For this review, take the finished solid that the model builds, in its own axes (mm). A direction names the side the tool comes from. Coordinates: 2 decimals unless noted, no trailing zeros. Order: outer loops, then holes, each group sorted by start corner. A loop starts at its lowest first (then second) coordinate and runs counter-clockwise, first axis right, second up. Notation, with made-up numbers: (69, -22) -> (120, -22) arc R16 ccw to (120, 6) -> close; hole circle Ø5 at (0.25, -6.5). An arc over 180 degrees is marked (long way). Write item = value, one per line. Start each with the question number.
1) Machinability: for faces 4 (the face through (41, 9, -107.95)), 5 (the face through (45, 53, -295.275)), 6 (the face through (2.053, 67.327, -201.314)), which of the approach directions +Z, -Z, +X, -X, +Y, -Y give a long, thin tool a straight path to every point of the face, cutting with its end or side? Answer none if there is none.
2) Consider section C-C on z = -123. Give the boundary of the cut face in (x, y) (3 decimals).
3) Insertion check: pin 1 Ø10 at (x, y) = (68, 130.5) entering from -Z; pin 2 Ø2.5 at (x, z) = (65.5, -294) entering from +Y (3 decimals); pin 3 Ø12 at (x, z) = (50.5, -200.5) entering from +Y (3 decimals). Each pin has a flat end and moves straight along its axis. Give the tip position at first contact, or say it passes through.
4) Consider section B-B on y = 42.5. Give the boundary of the cut face in (x, z) (3 decimals), and give its area (3 significant figures).
5) Draft analysis for pull direction Z (two halves, no side actions). For faces 1 (the face through (15, 18, -292.1)), 2 (the face through (44, 81, 0)), 3 (the face through (45, 0, -53)), state which applies: +Z half, -Z half, draft (parallel to the pull), parting line (faces both ways), or undercut.
6) Wall thickness on probe 1 along Z at (x, y) = (45.5, 101.5) (3 decimals); probe 2 along X at (y, z) = (128, -23.5); probe 3 along Z at (x, y) = (61, 137): over which ranges is each line inside the solid? List them lowest first. Write a range as [from, to].
7) Consider section D-D on y = 144.5. Give the boundary of the cut face in (x, z), and give its area (3 significant figures).
8) Consider section A-A on x = 44.45. Give the boundary of the cut face in (y, z) (3 decimals), and give its area (3 significant figures).
Autodesk Inventor part; units mm, degrees
ref_plane "YZ Plane" through (0, 0, 0) normal (1, 0, 0) x (0, 1, 0)
ref_plane "XZ Plane" through (0, 0, 0) normal (0, 1, 0) x (-1, 0, 0)
ref_plane "XY Plane" through (0, 0, 0) normal (0, 0, 1) x (1, 0, 0)
sketch "Sketch1" plane through (0, 0, 0) normal (0, 1, 0) x (-1, 0, 0)
  line L0 (0, 0) -> (-88.9, 0)
  line L1 (-88.9, 0) -> (-88.9, -292.1)
  line L2 (-88.9, -292.1) -> (0, -292.1)
  line L3 (0, -292.1) -> (0, 0)
  dimension "d2" = 88.9
  dimension "d3" = 292.1
extrude "Extrusion1" add sketch "Sketch1" along normal blind 165.1
sketch "Sketch2" plane through (88.9, 0, -292.1) normal (0, 0, -1) x (-1, 0, 0)
  line L0 (88.9, 165.1) -> (0, 165.1)
  line L1 (0, 0) -> (88.9, 0)
  line L2 (88.9, 0) -> (88.9, 165.1)
  line L3 (88.9, 165.1) -> (0, 165.1)
  line L4 (0, 165.1) -> (0, 0)
  circle A0 centre (44.45, 53.975) radius 44.45
  dimension "d6" = 44.45
  dimension "d7" = 88.9
  dimension "d8" = 53.975
extrude "Extrusion2" cut sketch "Sketch2" against normal blind 184.15 contours L2 A0 L4 L0 | L2 L1 L4 A0
sketch "Sketch3" plane through (44.45, 53.975, -292.1) normal (0, 0, -1) x (-1, 0, 0)
  line L0 (-44.3996, -53.975) -> (44.5004, -53.975)
  line L1 (44.5004, -53.975) -> (44.5004, 50.8)
  line L2 (44.5004, 50.8) -> (-44.3996, 50.8)
  line L3 (-44.3996, 50.8) -> (-44.3996, -53.975)
  point P0 (44.45, -53.975)
  dimension "d11" = 88.9
  dimension "d12" = 104.775
extrude "Extrusion3" add sketch "Sketch3" along normal blind 3.175
properties part number "compressor"
Answer sheet:
q1.face_4 = -Y
q1.face_5 = -Z, +X, -X, +Y, -Y
q1.face_6 = none
q2.outline = circle Ø88.9 at (44.45, 53.975)
q3.pin_1 = -107.95
q3.pin_2 = 104.775
q3.pin_3 = 98.425
q4.outline = (-0.05, -295.275) -> (88.85, -295.275) -> (88.85, -292.1) -> (87.393, -292.1) -> (87.393, -107.95) -> (88.9, -107.95) -> (88.9, 0) -> (0, 0) -> (0, -107.95) -> (1.507, -107.95) -> (1.507, -292.1) -> (-0.05, -292.1) -> close
q4.area = 25,700 mm2
q5.face_1 = undercut
q5.face_2 = +Z half
q5.face_3 = draft
q6.probe_1 = [-295.275, -292.1], [-107.95, 0]
q6.probe_2 = [0, 88.9]
q6.probe_3 = [-107.95, 0]
q7.outline = (0, -107.95) -> (88.9, -107.95) -> (88.9, 0) -> (0, 0) -> close
q7.area = 9,600 mm2
q8.outline = (0, -295.275) -> (104.775, -295.275) -> (104.775, -292.1) -> (98.425, -292.1) -> (98.425, -107.95) -> (165.1, -107.95) -> (165.1, 0) -> (0, 0) -> (0, -107.95) -> (9.525, -107.95) -> (9.525, -292.1) -> (0, -292.1) -> close
q8.area = 34,500 mm2
